from build123d import *

# Parameters (mm, degrees)
SKETCH001_R        = 1.6
POCKET_DEPTH       = 20.001
SKETCH003_W        = 22.2
SKETCH003_H        = 22.2
POCKET001_DEPTH    = 5.1
SKETCH004_R        = 2.9
POCKET002_DEPTH    = 3
SKETCH005_R        = 6
POCKET003_DEPTH    = 244.783506
POLARPATTERN_COUNT = 10


with BuildPart() as part:
    # Sketch → Revolution (revolve)
    with BuildSketch(Plane.XY):
        Polygon((8, 39), (8, 40), (10, 40), (10, 38.958768), (5, 33), (5, 16), (10, 16), (10, 1), (-10, 1), (-10, 16), (-5, 16), (-5, 33), (-10, 38.958768), (-10, 40), (-8, 40), (-8, 39), (-6.75, 37.510308), (6.75, 37.510308), align=None)
    revolve(axis=Axis((0, 0, 0), (1, 0, 0)))

    # Sketch001 (on Face7 of Revolution) → Pocket (cut, through all)
    with BuildSketch(Plane.YZ.offset(10)):
        with Locations((-7, 7)):
            Circle(SKETCH001_R)
        with Locations((7, 7)):
            Circle(SKETCH001_R)
        Polygon((-10.1, -7.393713), (0, 10.1), (10.1, -7.393713), align=None)
    extrude(amount=-POCKET_DEPTH, mode=Mode.SUBTRACT)

    # Sketch003 (on Face13 of Pocket) → Pocket001 (cut)
    with BuildSketch(Plane.YZ.offset(10)):
        Rectangle(SKETCH003_W, SKETCH003_H)
    extrude(amount=-POCKET001_DEPTH, mode=Mode.SUBTRACT)

    # Sketch004 (on Face27 of Pocket001) → Pocket002 (cut)
    with BuildSketch(Plane(origin=(-10, 0, 0), x_dir=(0, -1, 0), z_dir=(-1, 0, 0))):
        with Locations((-7, 7)):
            Circle(SKETCH004_R)
        with Locations((7, 7)):
            Circle(SKETCH004_R)
    extrude(amount=-POCKET002_DEPTH, mode=Mode.SUBTRACT)

    # Sketch005 (on Face9 of Pocket002) → Pocket003 (cut, through all)
    with BuildSketch(Plane.YZ.offset(5)):
        with Locations((0, 24)):
            Circle(SKETCH005_R)
    pocket003 = extrude(amount=-POCKET003_DEPTH, mode=Mode.SUBTRACT)

    # PolarPattern: Pocket003 ×10 about axis
    polarpattern_axis = Axis((5, 0, 0), (1, 0, 0))
    for i in range(1, POLARPATTERN_COUNT):
        add(pocket003.rotate(polarpattern_axis, i * 360 / POLARPATTERN_COUNT), mode=Mode.SUBTRACT)


solid = part.part
Could you check a few things on this model? Use its own coordinates, in mm. A direction names the side the tool comes from. Coordinates: 2 decimals unless noted, no trailing zeros. Answer in a Markdown table with one row per item. Add a question column.
(1) On a 3-axis mill with a long thin cutter (end or side, diameter ignored), from which of +Z, -Z, +X, -X, +Y, -Y can I reach the whole of each face in a straight line? I mean faces 1 (the face through (10, 38.3, -8.7)), 2 (the face through (-7, -8.25, 5.75)), 3 (the face through (4.9, -5, 3)), 4 (the face through (-2.446, 4.979, 1.476)). Say none if no direction works.
(2) I need wall thicknesses on L1, parallel to Z at x = -2.5, y = 22; L2, parallel to Z at x = 3, y = 16; L3, parallel to Y at x = -6, z = 7.5. Which ranges of each line are inside material? Lowest first, please.
(3) If we section it at A-A, the plane x = -3: State how many separate pieces and enclosed holes the cut face has, then the cut area to 3 significant figures.
(4) Will these pins go through, and if not, where does the flat tip stop? pin 1 (4 mm diameter, centred on y = 7, z = 7, fed in from -X); pin 2 (6 mm diameter, centred on x = 3, y = 19.5, fed in from -Z); pin 3 (4 mm diameter, centred on y = -7, z = 7, fed in from +X).
Results are:
| question | item | result |
|---|---|---|
| 1 | face 1 | +Z, -Z, +X, +Y, -Y |
| 1 | face 2 | -X |
| 1 | face 3 | +X |
| 1 | face 4 | +X, -X |
| 2 | L1 | z = -30.38 to -13.36, -1.47 to 1.47, 13.36 to 30.38 |
| 2 | L2 | z = -33.93 to -25.11, -13.72 to 13.72, 25.11 to 33.93 |
| 2 | L3 | y = -36.75 to -33.36, -14.13 to -8.52, -5.48 to -1.5, 1.5 to 5.48, 8.52 to 14.13, 33.36 to 36.75 |
| 3 | separate pieces | 1 |
| 3 | enclosed holes | 13 |
| 3 | area | 3,100 mm2 |
| 4 | pin 1 | stops at x = -7 |
| 4 | pin 2 | stops at z = -33.69 |
| 4 | pin 3 | stops at x = 4.9 |
